```python
from build123d import *

# Parameters (mm, degrees)
F1_DEPTH = 0.5
F2_DEPTH = 0.75


with BuildPart() as f1:
    # F0 (on Top) → F1 (new body)
    with BuildSketch(Plane.XY):
        with BuildLine():
            ThreePointArc((29.9959010885, -0.4959010884), (29.9989752546, -0.247959014), (30, 0))
            ThreePointArc((30, 0), (29.9989752546, 0.2479590141), (29.9959010885, 0.4959010885))
            ThreePointArc((29.9959010885, 0.4959010885), (29.9958671362, 0.4979505454), (29.9958330439, 0.5))
            ThreePointArc((29.9958330439, 0.5), (29.9957976483, 0.5021189497), (29.9957621031, 0.5042378969))
            Line((29.9957621031, 0.5042378969), (0.5042378969, 29.9957621031))
            ThreePointArc((0.5042378969, 29.9957621031), (0.5021189497, 29.9957976483), (0.5, 29.9958330439))
            ThreePointArc((0.5, 29.9958330439), (0.4979505454, 29.9958671362), (0.4959010885, 29.9959010885))
            ThreePointArc((0.4959010885, 29.9959010885), (0, 30), (-0.4959010885, 29.9959010885))
            ThreePointArc((-0.4959010885, 29.9959010885), (-0.4979505454, 29.9958671362), (-0.5, 29.9958330439))
            ThreePointArc((-0.5, 29.9958330439), (-0.5021189497, 29.9957976483), (-0.5042378969, 29.9957621031))
            Line((-0.5042378969, 29.9957621031), (-29.9957621031, 0.5042378969))
            ThreePointArc((-29.9957621031, 0.5042378969), (-29.9957976483, 0.5021189497), (-29.9958330439, 0.5))
            ThreePointArc((-29.9958330439, 0.5), (-29.9958671362, 0.4979505455), (-29.9959010885, 0.4959010886))
            ThreePointArc((-29.9959010885, 0.4959010886), (-30, 1e-10), (-29.9959010885, -0.4959010884))
            ThreePointArc((-29.9959010885, -0.4959010884), (-29.9958671362, -0.4979505453), (-29.9958330439, -0.4999999999))
            ThreePointArc((-29.9958330439, -0.4999999999), (-29.9957976483, -0.5021189497), (-29.9957621031, -0.5042378969))
            Line((-29.9957621031, -0.5042378969), (-0.5042378969, -29.9957621031))
            ThreePointArc((-0.5042378969, -29.9957621031), (-0.5021189497, -29.9957976483), (-0.5, -29.9958330439))
            ThreePointArc((-0.5, -29.9958330439), (-0.4979505454, -29.9958671362), (-0.4959010885, -29.9959010885))
            ThreePointArc((-0.4959010885, -29.9959010885), (1.6e-09, -30), (0.4959010917, -29.9959010884))
            ThreePointArc((0.4959010917, -29.9959010884), (0.497950547, -29.9958671362), (0.5, -29.9958330439))
            ThreePointArc((0.5, -29.9958330439), (0.5021189497, -29.9957976483), (0.5042378969, -29.9957621031))
            Line((0.5042378969, -29.9957621031), (29.9957621031, -0.5042378969))
            ThreePointArc((29.9957621031, -0.5042378969), (29.9957976483, -0.5021189497), (29.9958330439, -0.5))
            ThreePointArc((29.9958330439, -0.5), (29.9958671362, -0.4979505454), (29.9959010885, -0.4959010884))
        make_face()
        Polygon((-0.4999999985, -28.9999999984), (-6.8976368761, -22.6023631214), (-0.4999999992, -16.1435156014), align=None, mode=Mode.SUBTRACT)
        Polygon((-0.9606463591, -15.253539578), (-7.6035533893, -21.8964466082), (-14.1500740262, -15.349925972), align=None, mode=Mode.SUBTRACT)
        Polygon((-15.3535533902, -1.0606601714), (-15.3535533898, -14.1464466085), (-21.8964466089, -7.6035533901), align=None, mode=Mode.SUBTRACT)
        Polygon((-16.2388987995, -0.5), (-22.6041527374, -6.8958472617), (-28.9999999999, -0.4999999999), align=None, mode=Mode.SUBTRACT)
        Polygon((-1.1603910767, -14.5467157044), (-13.9276378166, -14.6364271465), (-7.4916261871, -8.2154805941), align=None, mode=Mode.SUBTRACT)
        Polygon((-8.1987320116, -7.5083747696), (-14.6464466094, -13.9409951753), (-14.6464466094, -1.0606601718), align=None, mode=Mode.SUBTRACT)
        Polygon((-6.783690857, -7.5092023618), (-0.5, -1.2402200376), (-0.4999999993, -13.7928932195), align=None, mode=Mode.SUBTRACT)
        Polygon((-13.7928932189, -0.5), (-1.1739120379, -0.5), (-7.4907965869, -6.8020966319), align=None, mode=Mode.SUBTRACT)
        Polygon((0.5, -16.2071067812), (6.8964466094, -22.6035533906), (0.5, -29), align=None, mode=Mode.SUBTRACT)
        Polygon((0.9467076968, -15.2396009156), (14.3584098275, -15.1415901725), (7.6035533906, -21.8964466094), align=None, mode=Mode.SUBTRACT)
        Polygon((14.0112935653, -14.4401090307), (1.0973812984, -14.5308510455), (7.5382237147, -8.0283846086), align=None, mode=Mode.SUBTRACT)
        Polygon((0.5, -13.7928932189), (0.5, -1.0568622983), (6.8983340381, -7.3945591808), align=None, mode=Mode.SUBTRACT)
        Polygon((14.7168418348, -0.7810836543), (14.7168418349, -13.7281676466), (8.2432305686, -7.3166324636), align=None, mode=Mode.SUBTRACT)
        Polygon((1.360599895, -0.5), (13.7928932189, -0.5), (7.6066937554, -6.6861994634), align=None, mode=Mode.SUBTRACT)
        Polygon((15.4256417891, -1.1327485702), (21.8964466095, -7.6035533905), (15.4256417891, -14.0743582109), align=None, mode=Mode.SUBTRACT)
        Polygon((29, -0.5), (22.6035533906, -6.8964466094), (16.2071067811, -0.5), align=None, mode=Mode.SUBTRACT)
        Polygon((-29, 0.5), (-22.6035533906, 6.8964466094), (-16.2071067813, 0.5), align=None, mode=Mode.SUBTRACT)
        Polygon((-21.8964466094, 7.6035533906), (-15.3535533906, 14.1464466094), (-15.3535533903, 1.0606601714), align=None, mode=Mode.SUBTRACT)
        Polygon((-13.7928932187, 0.5), (-7.4626086697, 6.8302845491), (-1.0717578841, 0.5000000001), align=None, mode=Mode.SUBTRACT)
        Polygon((-14.6464466094, 1.1001059941), (-14.6464466094, 13.9460410951), (-8.2084439991, 7.5690515803), align=None, mode=Mode.SUBTRACT)
        Polygon((-13.9325727794, 14.6465249656), (-1.1641236528, 14.6472290479), (-7.5026392249, 8.2782486645), align=None, mode=Mode.SUBTRACT)
        Polygon((-6.7550575733, 7.5378356455), (-0.5, 13.7928932188), (-0.5, 1.3427584231), align=None, mode=Mode.SUBTRACT)
        Polygon((-1.0606601718, 15.3535533906), (-14.1464466094, 15.3535533906), (-7.6035533906, 21.8964466094), align=None, mode=Mode.SUBTRACT)
        Polygon((-6.8964466094, 22.6035533906), (-0.5, 29), (-0.5, 16.2071067812), align=None, mode=Mode.SUBTRACT)
        Polygon((0.5000000005, 1.1699933855), (0.500000001, 13.7928932188), (6.8188461713, 7.4740470475), align=None, mode=Mode.SUBTRACT)
        Polygon((13.7928932184, 0.4999999994), (1.2443030111, 0.499999999), (7.5259499895, 6.7669432292), align=None, mode=Mode.SUBTRACT)
        Polygon((14.7168418348, 0.9902649463), (8.2338853191, 7.473221462), (14.7168418347, 13.941003014), align=None, mode=Mode.SUBTRACT)
        Polygon((14.0096987803, 14.6480657682), (7.5267815959, 8.1803251852), (1.0597551034, 14.6473516778), align=None, mode=Mode.SUBTRACT)
        Polygon((15.9857846309, 0.5000000004), (22.4619115095, 7.0380884906), (29, 0.5), align=None, mode=Mode.SUBTRACT)
        Polygon((15.4256417891, 1.1327485702), (15.4256417891, 14.074358211), (21.8964466094, 7.6035533906), align=None, mode=Mode.SUBTRACT)
        Polygon((1.0606601718, 15.3535533906), (7.6035533906, 21.8964466094), (14.1464466094, 15.3535533907), align=None, mode=Mode.SUBTRACT)
        Polygon((0.5, 16.3193509792), (0.5, 29), (6.825124286, 22.674875714), align=None, mode=Mode.SUBTRACT)
    extrude(amount=F1_DEPTH)

    # F0 (on Top) → F2 (join)
    with BuildSketch(Plane.XY):
        with BuildLine():
            ThreePointArc((0.5042378969, -29.9957621031), (21.2132034356, -21.2132034356), (29.9957621031, -0.5042378969))
            Line((29.9957621031, -0.5042378969), (0.5042378969, -29.9957621031))
        make_face()
        with BuildLine():
            Line((0.5042378969, 29.9957621031), (29.9957621031, 0.5042378969))
            ThreePointArc((29.9957621031, 0.5042378969), (21.2132034356, 21.2132034356), (0.5042378969, 29.9957621031))
        make_face()
        with BuildLine():
            Line((-29.9957621031, 0.5042378969), (-0.5042378969, 29.9957621031))
            ThreePointArc((-0.5042378969, 29.9957621031), (-21.2132034356, 21.2132034356), (-29.9957621031, 0.5042378969))
        make_face()
        with BuildLine():
            ThreePointArc((-29.9957621031, -0.5042378969), (-21.2132034356, -21.2132034356), (-0.5042378969, -29.9957621031))
            Line((-0.5042378969, -29.9957621031), (-29.9957621031, -0.5042378969))
        make_face()
    extrude(amount=F2_DEPTH)


solid = f1.part
```
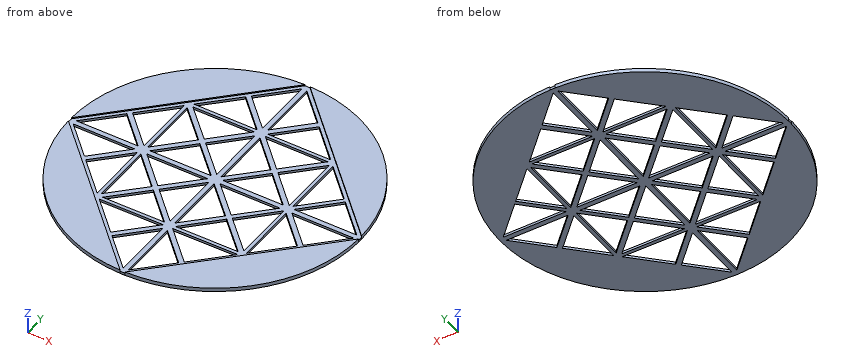
Check sheet for the modelled part. Datum: model origin and axes. Units: mm. Give positions to 0.01 mm unless a question says otherwise; leave off trailing zeros. Order: outer loops, then holes, each group sorted by start corner. A loop starts at its lowest first (then second) coordinate and runs counter-clockwise, first axis right, second up. Notation, with made-up numbers: M 77.5,12 L 130.5,12 A12 cw 130.5,27 Z; hole C -3,-19.75 d9. An arc over 180 degrees is marked long. Answer in a Markdown table with one row per item. Add a question column.
Q1. Sectioned sample at A-A, the plane y = 24.5. Record the boundary of the cut face in (x, z), and give its area (3 significant figures).
Q2. Gauge pin test, flat end, axial feed: pin 1 Ø4 at (x, y) = (15, -1) entering from +Z. Record the tip position at first contact, or that the pin passes through.
Q3. Sectioned sample at B-B, the plane x = 20. Record the boundary of the cut face in (y, z), and give its area (3 significant figures).
Q4. Sectioned sample at C-C, the plane z = 0.3. Count the separate pieces of the cut face and the enclosed holes in it, and give its area (3 significant figures).
Q5. Thickness scan on L1, parallel to Y at x = -18.5, z = 0.4; L2, parallel to X at y = -20, z = 0.45; L3, parallel to X at y = -16, z = 0.25. Record the ranges inside material, lowest first.
Verdict:
| question | item | result |
|---|---|---|
| 1 | outline | M -17.31,0 L -5,0 L -5,0.5 L -6,0.5 L -6,0.75 L -17.31,0.75 Z; M -0.5,0 L 0.5,0 L 0.5,0.5 L -0.5,0.5 Z; M 5,0 L 17.31,0 L 17.31,0.75 L 6,0.75 L 6,0.5 L 5,0.5 Z |
| 1 | area | 18.5 mm² |
| 2 | pin 1 | z = 0.5 |
| 3 | outline | M -22.36,0 L -9.5,0 L -9.5,0.5 L -10.5,0.5 L -10.5,0.75 L -22.36,0.75 Z; M -5.71,0 L -4.29,0 L -4.29,0.5 L -5.71,0.5 Z; M -0.5,0 L 0.5,0 L 0.5,0.5 L -0.5,0.5 Z; M 4.55,0 L 5.71,0 L 5.71,0.5 L 4.55,0.5 Z; M 9.5,0 L 22.36,0 L 22.36,0.75 L 10.5,0.75 L 10.5,0.5 L 9.5,0.5 Z |
| 3 | area | 20.6 mm² |
| 4 | separate pieces | 1 |
| 4 | enclosed holes | 32 |
| 4 | area | 1,510 mm² |
| 5 | L1 | -23.62 to -11, -4.21 to -2.77, -0.5 to 0.5, 2.79 to 4.21, 11 to 23.62 |
| 5 | L2 | -22.36 to -9.5, -5.71 to -4.32, -0.5 to 0.5, 4.29 to 5.71, 9.5 to 22.36 |
| 5 | L3 | -25.38 to -13.5, -1.71 to 1.71, 13.5 to 25.38 |
